from build123d import *

# Parameters (mm, degrees)
SKETCH1_R           = 1.524
BOSS_EXTRUDE1_DEPTH = 5.08
CHAMFER1_SIZE       = 1.27
CHAMFER1_SIZE2      = 0.340295474


with BuildPart() as part:
    # Sketch1 → Boss-Extrude1 (new body, symmetric)
    with BuildSketch(Plane(origin=(0, 0, 0), x_dir=(1, 0, 0), z_dir=(0, 1, 0))):
        Circle(SKETCH1_R)
    extrude(amount=BOSS_EXTRUDE1_DEPTH, both=True)

    # Chamfer1
    chamfer1_edges = [part.edges().sort_by_distance(p)[0] for p in [
        (-1.524, -5.08, 0),
    ]]
    chamfer1_side = [part.faces().sort_by_distance(p)[0] for p in [
        (-1.524, 0, 0),
    ]]
    chamfer(chamfer1_edges, length=CHAMFER1_SIZE, length2=CHAMFER1_SIZE2, reference=chamfer1_side[0])

    # Sketch2 → Revolve1 (revolve)
    with BuildSketch(Plane.XY):
        with BuildLine():
            Line((0, 5.08), (2.286, 5.08))
            Line((2.286, 5.08), (2.286, 5.842))
            ThreePointArc((2.286, 5.842), (2.137210245, 6.201210245), (1.778, 6.35))
            Line((1.778, 6.35), (0, 6.35))
            Line((0, 6.35), (0, 5.08))
        make_face()
    revolve(axis=Axis((0, 5.08, 0), (0, 1, 0)))


solid = part.part
The model under review builds one solid part; all positions refer to its coordinate system, in mm. A direction names the side the tool comes from. Coordinates: 2 decimals unless noted, no trailing zeros. Loops run counter-clockwise (first coordinate to the right, second up) from the corner with the lowest first, then second, coordinate; pieces in that order, holes last.
(1) Insertion check: P1, Ø1.5, axis at y = -1.5, z = 1, coming from the -X side; P2, Ø1.5, axis at y = 4.5, z = 0.5, coming from the +X side. Each pin has a flat end and moves straight along its axis. Give the tip position at first contact, or say it passes through.
Determined:
P1: stops at x = -1.5
P2: stops at x = 2.29
(2) Consider section C-C, the plane y = 5.25. Give the boundary of the cut face in (x, z), plus the area to 3 significant figures.
Determined:
outline: circle Ø4.57 at (0, 0)
area: 16.4 mm2
(3) Wall thickness on L1, parallel to X at y = -3, z = 0; L2, parallel to X at y = 5.25, z = -0.1; L3, parallel to Y at x = -0.95, z = 1.3: over which ranges is each line inside the solid? List them lowest first.
Determined:
L1: x = -1.52 to 1.52
L2: x = -2.28 to 2.28
L3: y = 5.08 to 6.35
(4) Consider section B-B, the plane x = 0. Give the boundary of the cut face in (y, z), plus the area to 3 significant figures.
Determined:
outline: (-5.08, -1.18) - (-3.81, -1.52) - (5.08, -1.52) - (5.08, -2.29) - (5.84, -2.29) arc R0.51 ccw to (6.35, -1.78) - (6.35, 1.78) arc R0.51 ccw to (5.84, 2.29) - (5.08, 2.29) - (5.08, 1.52) - (-3.81, 1.52) - (-5.08, 1.18) - close
area: 36.2 mm2
(5) Tool access review of faces 1 (the cylindrical face through (-0.5, 5.47, 2.23)), 2 (the flat face through (0, 5.08, -2)): name each direction out of +Z, -Z, +X, -X, +Y, -Y from which nothing blocks a thin tool from reaching the whole face with its end or side.
Determined:
face 1: +Y, -Y
face 2: -Y
(6) Consider section A-A, the plane z = 0. Give the boundary of the cut face in (x, y).
Determined:
outline: (-2.29, 5.08) - (-1.52, 5.08) - (-1.52, -3.81) - (-1.18, -5.08) - (1.18, -5.08) - (1.52, -3.81) - (1.52, 5.08) - (2.29, 5.08) - (2.29, 5.84) arc R0.51 ccw to (1.78, 6.35) - (-1.78, 6.35) arc R0.51 ccw to (-2.29, 5.84) - close
(7) Consider section D-D, the plane y = 2.25. Give the boundary of the cut face in (x, z).
Determined:
outline: circle Ø3.05 at (0, 0)
